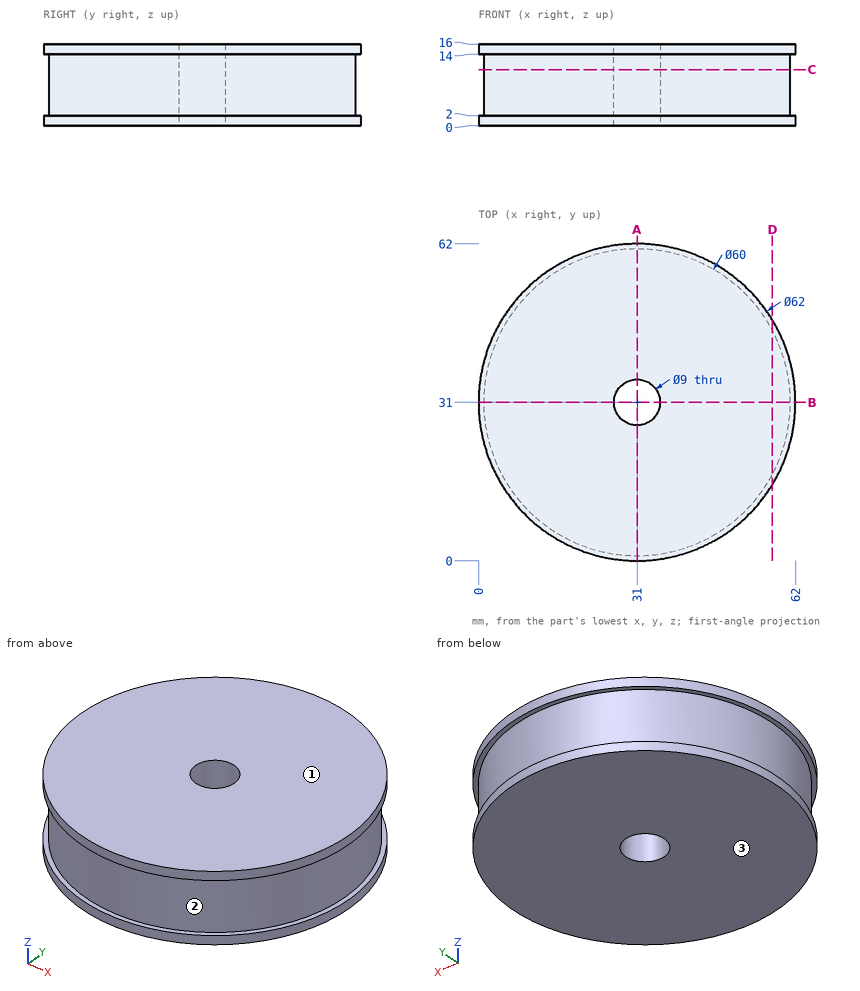
Job drawing, mm, ordinate dimensions from the low corner. One solid piece. Round coordinates to 2 decimals unless told otherwise and drop trailing zeros. Loops run counter-clockwise (first coordinate to the right, second up) from the corner with the lowest first, then second, coordinate; pieces in that order, holes last. Notation, with made-up numbers: (81, 0.5) -> (119, 0.5) arc R21 ccw to (119, 38.5) -> close; hole circle Ø11 at (-36.5, 5). An arc over 180 degrees is marked (long way). Use CSV: the item, a comma, the result in double quotes. Start each with the question number.
Q1. Saw through at D-D on x = 57.5. Give the cut face in (y, z).
Q2. Flat gauge pins, fed straight in: pin 1 Ø18.5 at (x, y) = (42, 29) entering from -Z; pin 2 Ø8 at (y, z) = (34.5, 9) entering from +X; pin 3 Ø8 at (x, z) = (34.5, 12) entering from +Y; pin 4 Ø5 at (x, z) = (49, 2) entering from -Y. Where does each tip first touch, or does it go through?
Q3. Drill centre lines: L1, parallel to Z at x = 50, y = 7; L2, parallel to Y at x = 31, z = 10; L3, parallel to Y at x = 30, z = 5.25. Where is each one in solid material? Low to high.
Q4. Saw through at C-C on z = 11. Give the cut face in (x, y).
Q5. Mould opens along Z. For the marked faces 1, 2 and 3 say: +Z half, -Z half, draft (parallel to the pull), parting line (faces both ways), or undercut.
Q6. Saw through at A-A on x = 31. Give the cut face in (y, z).
Solutions:
1,outline,"(14.91, 0) -> (47.09, 0) -> (47.09, 2) -> (45.06, 2) -> (45.06, 14) -> (47.09, 14) -> (47.09, 16) -> (14.91, 16) -> (14.91, 14) -> (16.94, 14) -> (16.94, 2) -> (14.91, 2) -> close"
2,pin 1,"stops at z = 0"
2,pin 2,"stops at x = 61"
2,pin 3,"stops at y = 62"
2,pin 4,"stops at y = 4.15"
3,L1,"z = 0 to 2, 14 to 16"
3,L2,"y = 1 to 26.5, 35.5 to 61"
3,L3,"y = 1.02 to 26.61, 35.39 to 60.98"
4,outline,"circle Ø60 at (31, 31); hole circle Ø9 at (31, 31)"
5,face 1,"+Z half"
5,face 2,"undercut"
5,face 3,"-Z half"
6,outline,"(0, 0) -> (26.5, 0) -> (26.5, 16) -> (0, 16) -> (0, 14) -> (1, 14) -> (1, 2) -> (0, 2) -> close; (35.5, 0) -> (62, 0) -> (62, 2) -> (61, 2) -> (61, 14) -> (62, 14) -> (62, 16) -> (35.5, 16) -> close"
